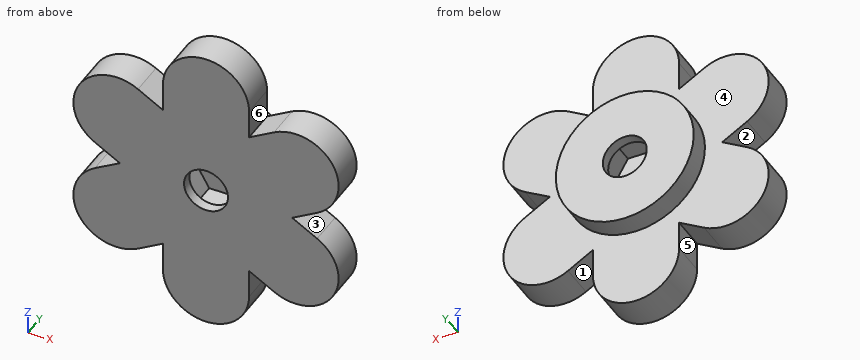
```python
from build123d import *

# Parameters (mm, degrees)
SKETCH1_R           = 8
BOSS_EXTRUDE1_DEPTH = 6.5
CUT_EXTRUDE1_START  = 1.2
CUT_EXTRUDE1_DEPTH  = 4.1
CUT_EXTRUDE2_REACH  = 15.048
SKETCH5_R           = 2.55
BOSS_EXTRUDE4_DEPTH = 4
CIRPATTERN1_COUNT   = 6


with BuildPart() as part:
    # Sketch1 → Boss-Extrude1 (new body)
    with BuildSketch(Plane(origin=(0, 0, 0), x_dir=(1, 0, 0), z_dir=(0, 1, 0))):
        with Locations(Location((0, 0, 0), (0, 0, 90))):
            Circle(SKETCH1_R)
    extrude(amount=BOSS_EXTRUDE1_DEPTH)

    # Sketch4 → Cut-Extrude1 (cut)
    with BuildSketch(Plane(origin=(0, 0, 0), x_dir=(1, 0, 0), z_dir=(0, 1, 0)).offset(CUT_EXTRUDE1_START)):
        Polygon((4.792007234, 0), (2.396003617, 4.15), (-2.396003617, 4.15), (-4.792007234, 0), (-2.396003617, -4.15), (2.396003617, -4.15), align=None)
    extrude(amount=CUT_EXTRUDE1_DEPTH, mode=Mode.SUBTRACT)

    # Cut-Extrude2: up to this face of the body (flat: up to its plane)
    cut_extrude2_end = Plane(part.part.faces().sort_by_distance((0, 6.5, 0))[0])
    # Sketch5 → Cut-Extrude2 (cut, up to the picked face)
    with BuildSketch(Plane(origin=(0, 0, 0), x_dir=(1, 0, 0), z_dir=(0, 1, 0)), mode=Mode.PRIVATE) as cut_extrude2_sk1:
        with Locations(Location((0, 0, 0), (0, 0, 90))):
            Circle(SKETCH5_R)
    cut_extrude2_tool1 = split(extrude(cut_extrude2_sk1.sketch, amount=CUT_EXTRUDE2_REACH, mode=Mode.PRIVATE), bisect_by=cut_extrude2_end, keep=Keep.BOTH, mode=Mode.PRIVATE)
    add(cut_extrude2_tool1.solids().sort_by(Axis((0, 0, 0), (0, 1, 0)))[0], mode=Mode.SUBTRACT)

    # Sketch6 → Boss-Extrude4 (add)
    with BuildSketch(Plane(origin=(0, 0, 0), x_dir=(1, 0, 0), z_dir=(0, 1, 0))):
        with BuildLine():
            Line((-5, 12), (-5, 6.244997998))
            ThreePointArc((-5, 6.244997998), (0, 8), (5, 6.244997998))
            Line((5, 6.244997998), (5, 12))
            ThreePointArc((5, 12), (0, 17), (-5, 12))
        make_face()
    boss_extrude4 = extrude(amount=BOSS_EXTRUDE4_DEPTH)

    # CirPattern1: Boss-Extrude4 ×6 about axis
    cirpattern1_axis = Axis((0, 0, 0), (0, 1, 0))
    for i in range(1, CIRPATTERN1_COUNT):
        add(boss_extrude4.rotate(cirpattern1_axis, i * 360 / CIRPATTERN1_COUNT))


solid = part.part
```
Build history of the part. All positions in model axes, mm. Face numbers are marked on the shaded views. A direction names the side the tool comes from. Round coordinates to 2 decimals unless told otherwise and drop trailing zeros. Write each loop counter-clockwise with the first axis right and the second up, starting at its lowest first coordinate (ties: lowest second). Pieces come first, ordered by that corner, then holes.
1) Band-saw the part on D-D, the plane z = -12.5. List the corners of the cut face in (x, y).
2) Mould opens along X. For the marked faces 1, 2 and 3 say: +X half, -X half, draft (parallel to the pull), parting line (faces both ways), or undercut.
3) Drill centre lines: probe 1 along X at (y, z) = (6.1, 0); probe 2 along Y at (x, z) = (12, 4.5); probe 3 along X at (y, z) = (3.5, -12). Where is each one in solid material? Low to high.
4) Pin check, flat tips, straight feed: pin 1 (1.5 mm diameter, centred on y = 4, z = -4, fed in from -X); pin 2 (8 mm diameter, centred on x = 10, z = -9.5, fed in from +Y); pin 3 (2 mm diameter, centred on y = 6, z = -1, fed in from -X); pin 4 (4.5 mm diameter, centred on x = 0, z = 0, fed in from +Y). Stop position of each tip, or through.
5) 3-axis set-ups, long thin cutter, end or side, ignore diameter. For the marked faces 4, 5 and 6: which of +Z, -Z, +X, -X, +Y, -Y reach the whole face in a straight line?
6) Band-saw the part on A-A, the plane y = 3.25. List the corners of the cut face in (x, z), and give its area (3 significant figures).
7) Band-saw the part on C-C, the plane y = 5.75. List the corners of the cut face in (x, z), and give its area (3 significant figures).
8) Band-saw the part on B-B, the plane x = 6.5. List the corners of the cut face in (y, z), and give its area (3 significant figures).
Ans:
1. outline: (-4.97, 0) - (4.97, 0) - (4.97, 4) - (-4.97, 4) - close
2. face 1: undercut
2. face 2: -X half
2. face 3: +X half
3. probe 1: x = -8 to -2.55, 2.55 to 8
3. probe 2: y = 0 to 4
3. probe 3: x = -5 to 5
4. pin 1: stops at x = -15.23
4. pin 2: stops at y = 4
4. pin 3: stops at x = -8
4. pin 4: passes through
5. face 4: +Y
5. face 5: -Z, +Y, -Y
5. face 6: +Z, +Y, -Y
6. outline: (-12.89, -1.67) arc R5 ccw to (-7.89, -10.33) - (-5, -8.66) - (-5, -12) arc R5 ccw to (5, -12) - (5, -8.66) - (7.89, -10.33) arc R5 ccw to (12.89, -1.67) - (10, 0) - (12.89, 1.67) arc R5 ccw to (7.89, 10.33) - (5, 8.66) - (5, 12) arc R5 ccw to (-5, 12) - (-5, 8.66) - (-7.89, 10.33) arc R5 ccw to (-12.89, 1.67) - (-10, 0) - close; hole (-4.79, 0) - (-2.4, -4.15) - (2.4, -4.15) - (4.79, 0) - (2.4, 4.15) - (-2.4, 4.15) - close
6. area: 636 mm2
7. outline: circle Ø16 at (0, 0); hole circle Ø5.1 at (0, 0)
7. area: 181 mm2
8. outline: (0, -9.53) - (4, -9.53) - (4, -4.66) - (6.5, -4.66) - (6.5, 4.66) - (4, 4.66) - (4, 9.53) - (0, 9.53) - close
8. area: 99.5 mm2
